Design review of the part shown in the three views and the two pictorial views. Dimensions are in mm from the part's minimum x, y and z. A direction names the side the tool comes from. Give positions to 0.01 mm unless a question says otherwise; leave off trailing zeros. Order: outer loops, then holes, each group sorted by start corner. A loop starts at its lowest first (then second) coordinate and runs counter-clockwise, first axis right, second up.
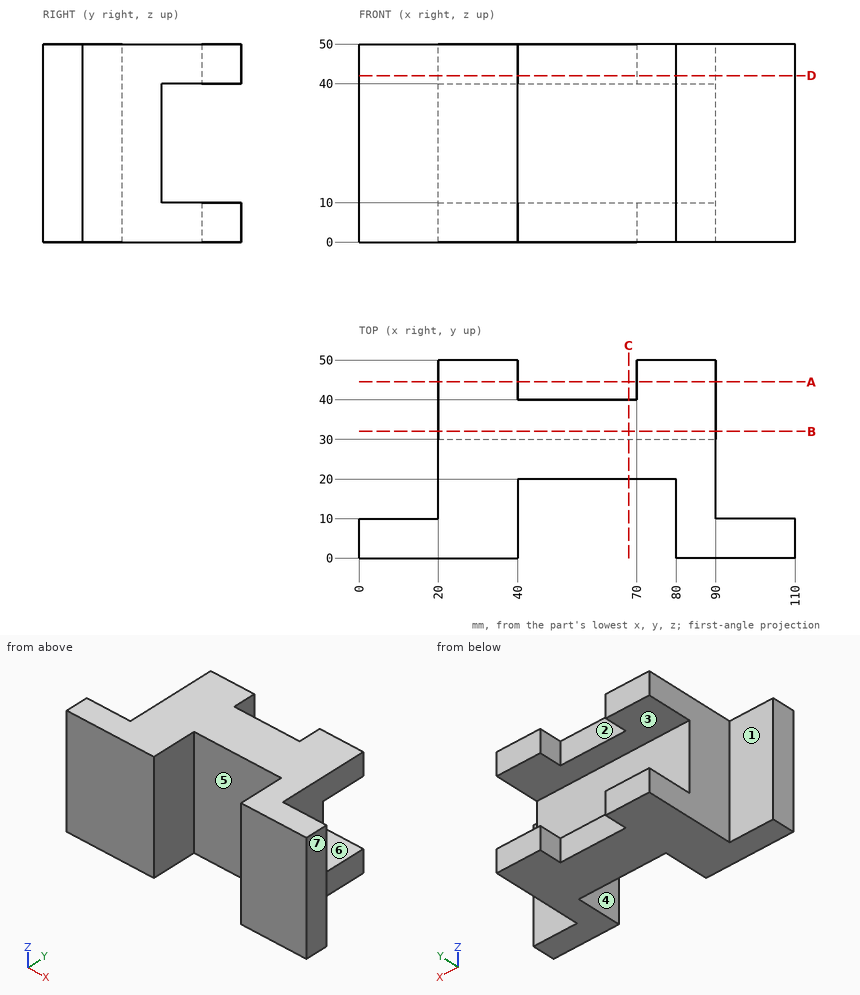
1) We need section C-C on x = 68. Give the boundary of the cut face in (y, z).
Answer sheet:
outline: (20, 0) - (40, 0) - (40, 10) - (30, 10) - (30, 40) - (40, 40) - (40, 50) - (20, 50) - close
2) We need section A-A on y = 44.5. Give the boundary of the cut face in (x, z), then the cut area to 3 significant figures.
Answer sheet:
outline: (20, 0) - (40, 0) - (40, 10) - (20, 10) - close; (20, 40) - (40, 40) - (40, 50) - (20, 50) - close; (70, 0) - (90, 0) - (90, 10) - (70, 10) - close; (70, 40) - (90, 40) - (90, 50) - (70, 50) - close
area: 800 mm2
3) To check wall thickness, follow line 1 (Z direction, x = 73, y = 35); line 2 (X direction, y = 12.5, z = 34.5); line 3 (X direction, y = 6.5, z = 12). State the ranges of each line that lie inside material, in increasing order.
Answer sheet:
line 1: z = 0 to 10, 40 to 50
line 2: x = 20 to 40, 80 to 90
line 3: x = 0 to 40, 80 to 110
4) Tool access review of the marked faces 1, 2, 3 and 4: name each direction out of +Z, -Z, +X, -X, +Y, -Y from which nothing blocks a thin tool from reaching the whole face with its end or side.
Answer sheet:
face 1: +Z, -Z, -X, +Y
face 2: +Z, -Z, +Y
face 3: +X, -X, +Y
face 4: +Z, -Z, -Y
5) We need section B-B on y = 32. Give the boundary of the cut face in (x, z).
Answer sheet:
outline: (20, 0) - (90, 0) - (90, 10) - (20, 10) - close; (20, 40) - (90, 40) - (90, 50) - (20, 50) - close
6) Draft analysis for pull direction X (two halves, no side actions). For the marked faces 5, 6 and 7, state which applies: +X half, -X half, draft (parallel to the pull), parting line (faces both ways), or undercut.
Answer sheet:
face 5: undercut
face 6: draft
face 7: +X half
7) Clearance check with flat-ended pins moving along their axes: pin 1 (12 mm diameter, centred on x = 64.5, z = 33, fed in from -Y); pin 2 (4 mm diameter, centred on y = 14.5, z = 14.5, fed in from -X); pin 3 (11 mm diameter, centred on x = 51, z = 44.5, fed in from +Y). State where each tip first meets the part, or that it passes through.
Answer sheet:
pin 1: stops at y = 20
pin 2: stops at x = 20
pin 3: stops at y = 40
8) We need section D-D on z = 42. Give the boundary of the cut face in (x, y), then the cut area to 3 significant figures.
Answer sheet:
outline: (0, 0) - (40, 0) - (40, 20) - (80, 20) - (80, 0) - (110, 0) - (110, 10) - (90, 10) - (90, 50) - (70, 50) - (70, 40) - (40, 40) - (40, 50) - (20, 50) - (20, 10) - (0, 10) - close
area: 2,800 mm2
